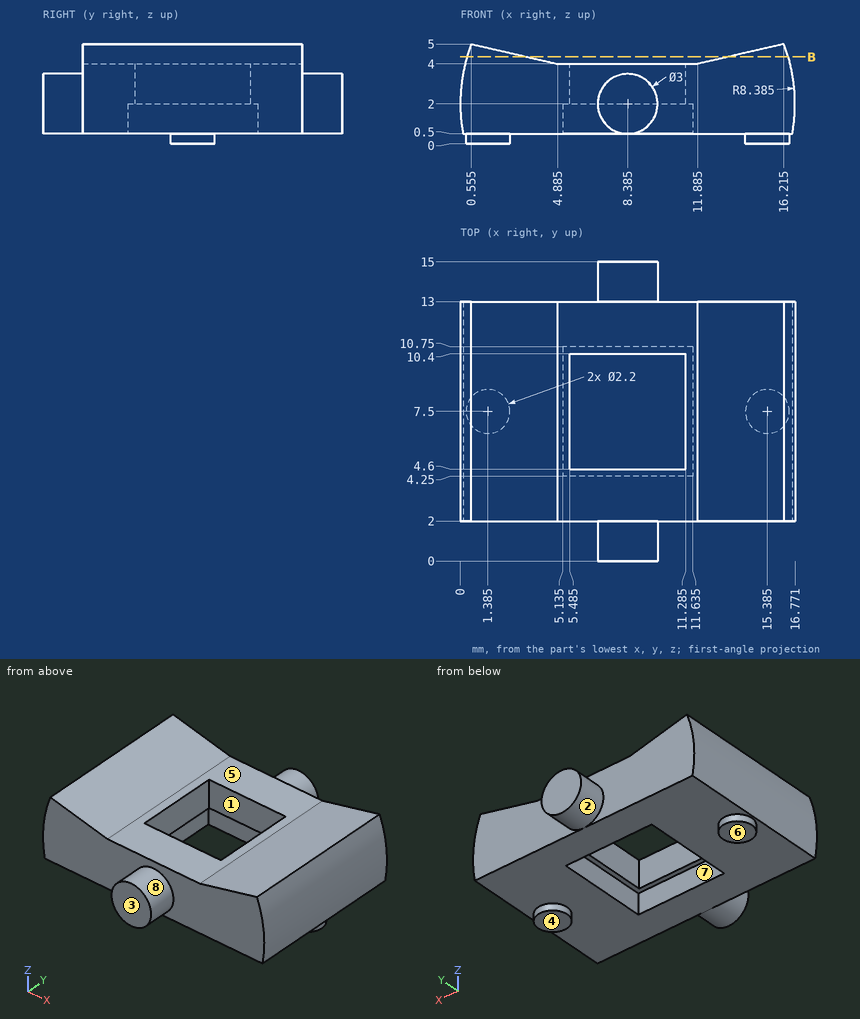
Here's the drawing with two shaded views (mm, measured from the low corner). I have some questions. A direction names the side the tool comes from. Give positions to 0.01 mm unless a question says otherwise; leave off trailing zeros. Write each loop counter-clockwise with the first axis right and the second up, starting at its lowest first coordinate (ties: lowest second). Pieces come first, ordered by that corner, then holes. Notation, with made-up numbers: (28, -20) -> (40, -20) arc R22 ccw to (40, -13) -> close; hole circle Ø10 at (-16.5, 17). An arc over 180 degrees is marked (long way). One line per item, written item: value.
Q1. Imagine slicing it at B-B on z = 4.35. Please give me the cut outline in (x, y) (1 decimal).
Results found:
outline: (0.3, 2) -> (3.4, 2) -> (3.4, 13) -> (0.3, 13) -> close; (13.4, 2) -> (16.4, 2) -> (16.4, 13) -> (13.4, 13) -> close
Q2. Which directions (+Z, -Z, +X, -X, +Y, -Y) give clear straight access to the entire face, cutting with the end or side of a thin tool? Please do the marked faces 1, 2, 3, 4 and 5.
Results found:
face 1: +Z, -Z
face 2: +Y
face 3: +Z, -Z, +X, -X, -Y
face 4: -Z, +X, -X, +Y, -Y
face 5: +Z, +Y, -Y
Q3. We'd pull the mould along X, two halves only. Please class the marked faces 6, 7 and 8: +X half, -X half, draft (parallel to the pull), parting line (faces both ways), or undercut.
Results found:
face 6: draft
face 7: undercut
face 8: parting line
Q4. Please list where these lines run through material, in increasing order: line 1 (Y direction, x = 6.25, z = 0.85); line 2 (Y direction, x = 9.5, z = 2.8); line 3 (Y direction, x = 3.25, z = 4.1). Write a range as [from, to].
Results found:
line 1: y = [2, 4.25], [10.75, 13]
line 2: y = [0, 4.6], [10.4, 15]
line 3: y = [2, 13]
Q5. For P1, Ø7.5, axis at x = 7, y = 6.5, coming from the +Z side; P2, Ø1.5, axis at y = 10, z = 3.5, coming from the -X side; P3, Ø2.5, axis at x = 12, z = 2.5, coming from the -Y side, each with a flat end and sliding along its axis, tell me the tip position at first contact or that it passes through.
Results found:
P1: stops at z = 4.38
P2: stops at x = 0.03
P3: stops at y = 2
